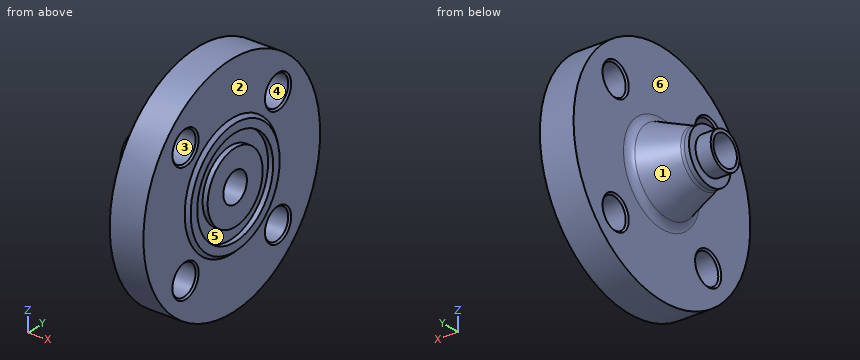
from build123d import *

# Parameters (mm, degrees)
SKETCH_3_R                           = 9.000000000000004
CUT_EXTRUDE_1_DEPTH                  = 112.43944544011336
CHAMFER_1_SIZE                       = 1
PATTERN_CIRCULAR_1_COUNT             = 4
CHAMFER_1_OF_PATTERN_CIRCULAR_1_SIZE = 1


with BuildPart() as part:
    # Эскиз1 → Повернуть1 (revolve)
    with BuildSketch(Plane.XY):
        with BuildLine():
            Line((3.06e-15, 9), (-59.50000000000001, 8.999999999999993))
            Line((-59.50000000000001, 8.999999999999993), (-59.50000000000001, 10.999999999999996))
            Line((-59.50000000000001, 10.999999999999996), (-50.5, 10.999999999999995))
            Line((-50.5, 10.999999999999995), (-47.09683777000456, 15.860219355388013))
            Line((-47.09683777000456, 15.860219355388013), (-25.126967032920497, 24.736623311378192))
            ThreePointArc((-25.126967032920497, 24.736623311378192), (-22.85481213722481, 26.576578066858403), (-22.000000000000007, 29.372542584212177))
            Line((-22.000000000000007, 29.372542584212177), (-22.000000000000007, 67.5))
            Line((-22.000000000000007, 67.5), (-2.0000000000000053, 67.5))
            Line((-2.0000000000000053, 67.5), (-2.0000000000000004, 36.00000000000003))
            Line((-2.0000000000000004, 36.00000000000003), (-6.7e-16, 34))
            Line((-6.7e-16, 34), (6.1e-16, 29))
            Line((6.1e-16, 29), (-2.999999999999999, 29))
            Line((-2.999999999999999, 29), (-2.9999999999999982, 21))
            Line((-2.9999999999999982, 21), (1.73e-15, 21))
            Line((1.73e-15, 21), (3.06e-15, 9))
        make_face()
    revolve(axis=Axis((0, 0, 0), (-1, -1.2e-16, 0)))

    # Эскиз2 → Повернуть2 (revolve)
    with BuildSketch(Plane.XY, mode=Mode.PRIVATE) as revolve_2_sk:
        with BuildLine():
            Line((-47.09683777000456, 15.86021935538801), (-50.5, 10.999999999999991))
            Line((-50.5, 10.999999999999991), (-50.5, 15.999999999999993))
            Line((-50.5, 15.999999999999993), (-47.722770079851955, 15.999999999999993))
            ThreePointArc((-47.722770079851955, 15.999999999999993), (-46.76872510296925, 16.09186408276167), (-45.849737112772424, 16.364080727166044))
            Line((-45.849737112772424, 16.364080727166044), (-47.09683777000456, 15.86021935538801))
        make_face()
    revolve(revolve_2_sk.sketch.rotate(Axis((0, 0, 0), (-1, 0, 0)), 90), axis=Axis((0, 0, 0), (-1, 0, 0)))

    # Эскиз3 → Вырез-Вытянуть1 (cut, through all)
    with BuildSketch(Plane(origin=(-1.9999999999999962, -2.4e-16, 0), x_dir=(0, 0, -1), z_dir=(1, 1.2e-16, 0))):
        with Locations(Location((35.35533905932718, 35.35533905932757, 0), (0, 0, 90))):
            Circle(SKETCH_3_R)
    cut_extrude_1 = extrude(amount=-CUT_EXTRUDE_1_DEPTH, mode=Mode.SUBTRACT)

    # Фаска1
    chamfer_1_edges = [part.edges().sort_by_distance(p)[0] for p in [
        (-22.000000000000007, 26.355339059327566, -35.35533905932718),
        (-1.9999999999999996, 26.355339059327566, -35.35533905932718),
    ]]
    chamfer(chamfer_1_edges, length=CHAMFER_1_SIZE)

    # Круговой массив1: Вырез-Вытянуть1 ×4 about axis
    pattern_circular_1_axis = Axis((0, 6.014e-14, 6.245e-14), (1, 0, 0))
    for i in range(1, PATTERN_CIRCULAR_1_COUNT):
        add(cut_extrude_1.rotate(pattern_circular_1_axis, i * 360 / PATTERN_CIRCULAR_1_COUNT), mode=Mode.SUBTRACT)

    # Фаска1 of Круговой массив1
    chamfer_1_of_pattern_circular_1_edges = [part.edges().sort_by_distance(p)[0] for p in [
        (-22.000000000000007, 35.3553390593273, 26.355339059327566),
        (-1.9999999999999996, 35.3553390593273, 26.355339059327566),
        (-22.000000000000007, -26.35533905932744, 35.35533905932731),
        (-1.9999999999999996, -26.35533905932744, 35.35533905932731),
        (-22.000000000000007, -35.355339059327186, -26.355339059327434),
        (-1.9999999999999996, -35.355339059327186, -26.355339059327434),
    ]]
    chamfer(chamfer_1_of_pattern_circular_1_edges, length=CHAMFER_1_OF_PATTERN_CIRCULAR_1_SIZE)


solid = part.part
The listing builds one solid part. Answer for the finished solid, in the listing's coordinates (mm). Face numbers are marked on the shaded views. A direction names the side the tool comes from. Give positions to 0.01 mm unless a question says otherwise; leave off trailing zeros. Write each loop counter-clockwise with the first axis right and the second up, starting at its lowest first coordinate (ties: lowest second). Pieces come first, ordered by that corner, then holes. Notation, with made-up numbers: (58, -20.75) -> (107, -20.75) arc R18 cw to (107, -10.75) -> close; hole circle Ø7 at (29, 67). An arc over 180 degrees is marked (long way). One line per question, with ' | ' between items. Start each with the question number.
1. For a pull along Z with two mould halves and no side action, classify the marked faces 1, 2 and 3 as pulls with the +Z half, pulls with the -Z half, needs draft (parallel to the pull), parting line crosses it, or undercut.
2. Given pin 1 Ø20.5 at (y, z) = (35.36, -35.36) entering from -X; pin 2 Ø4 at (x, z) = (-21.5, 48.5) entering from +Y; pin 3 Ø4 at (y, z) = (23, 37.5) entering from +X, each flat-ended and moving along its own axis, determine where each tip first touches the part or whether it passes through.
3. Section C-C (x = -56) is taken. Determine the outline of the cut face in (y, z).
4. Section D-D (z = 54) is taken. Determine the outline of the cut face in (x, y).
5. Find the intervals of material crossed by probe 1 along Y at (x, z) = (-14.5, 32.5); probe 2 along Z at (x, y) = (-0.65, 0); probe 3 along X at (y, z) = (-25, 48), in increasing order.
6. For the marked faces 4, 5 and 6, determine the directions among +Z, -Z, +X, -X, +Y, -Y from which every point of the face is accessible in a straight line to the end or side of a thin tool.
Response values:
1) face 1: parting line crosses it | face 2: needs draft | face 3: undercut
2) pin 1: x = -22 | pin 2: y = 48.93 | pin 3: x = -2
3) outline: circle Ø22 at (0, 0); hole circle Ø18 at (0, 0)
4) outline: (-22, -40.5) -> (-2, -40.5) -> (-2, 40.5) -> (-22, 40.5) -> close
5) probe 1: -59.16 to -43.89, -26.82 to 26.82, 43.89 to 59.16 | probe 2: -34.65 to -29, -21 to -9, 9 to 21, 29 to 34.65 | probe 3: -22 to -2
6) face 4: +X, -X | face 5: +X | face 6: -X
